Here's the drawing with two shaded views (mm, measured from the low corner). I have some questions. A direction names the side the tool comes from. Coordinates: 2 decimals unless noted, no trailing zeros. Order: outer loops, then holes, each group sorted by start corner. A loop starts at its lowest first (then second) coordinate and runs counter-clockwise, first axis right, second up. Notation, with made-up numbers: (-29.5, -35.75) -> (-23.5, -35.75) arc R31 cw to (-23.5, -4.75) -> close; hole circle Ø5 at (61.5, 20.25). An arc over 180 degrees is marked (long way). One line per item, written item: value. Start each with the question number.
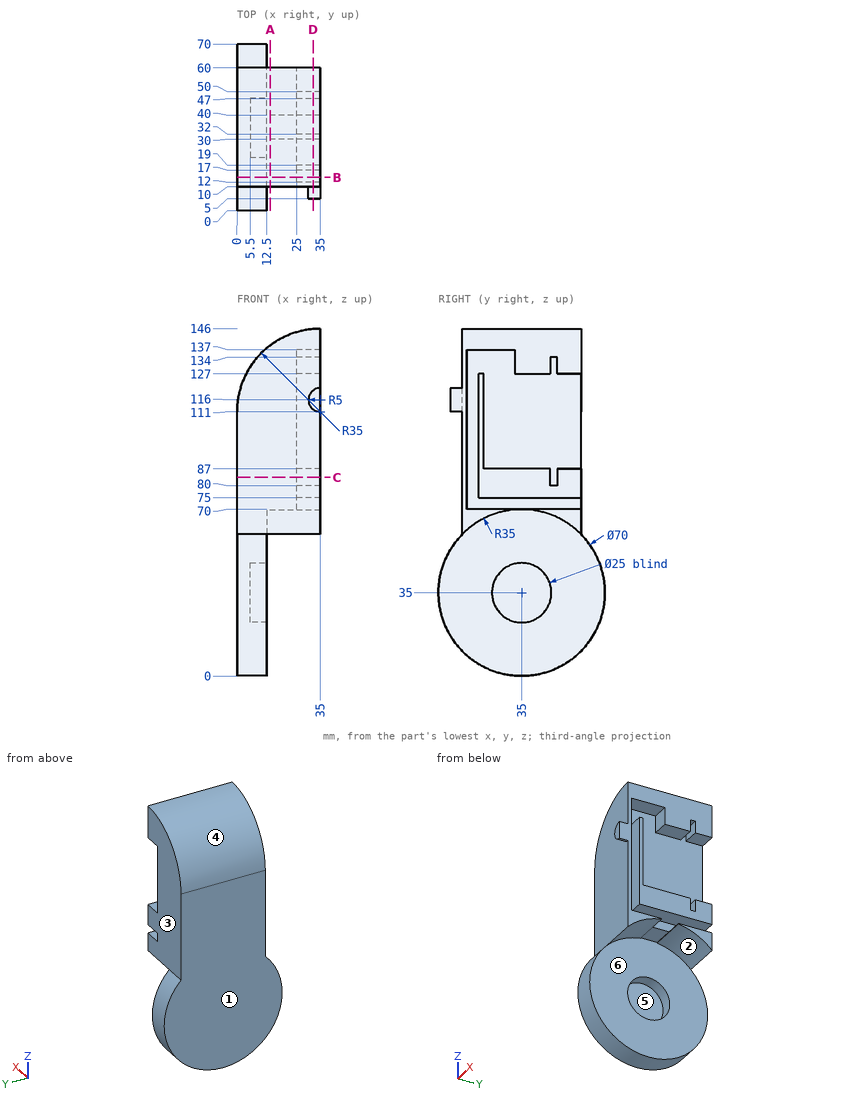
Q1. Imagine slicing it at C-C (z = 83.5). Write out the boundary of the cut face in (x, y), plus the area to 3 significant figures.
Q2. Imagine slicing it at A-A (x = 14). Write out the boundary of the cut face in (y, z), plus the area to 3 significant figures.
Q3. Imagine slicing it at B-B (y = 14). Write out the boundary of the cut face in (x, z), plus the area to 3 significant figures.
Q4. I need wall thicknesses on line 1 (Y direction, x = 33, z = 86.5); line 2 (Y direction, x = 31, z = 128); line 3 (Z direction, x = 33, y = 45). Which ranges of each line are inside material? Lowest first, please.
Q5. For P1, Ø3.5, axis at x = 29.5, z = 129, coming from the +Y side; P2, Ø5, axis at x = 28.5, z = 108, coming from the +Y side; P3, Ø1.5, axis at x = 31.5, z = 116, coming from the -Y side; P4, Ø12, axis at x = 20.5, z = 33.5, coming from the -Y side, each with a flat end and sliding along its axis, tell me the tip position at first contact or that it passes through.
Q6. For the marked faces 1, 2 and 3, which set-ups out of +Z, -Z, +X, -X, +Y, -Y let a thin tool reach every point of the face, with its end or its side?
Q7. If we mould it in two halves opening along Z, with no side actions, what happens to the marked faces 4, 5 and 6? For each: +Z half, -Z half, draft (parallel to the pull), parting line (faces both ways), or undercut.
Q8. Imagine slicing it at D-D (x = 32). Count the separate pieces of the cut face and the enclosed holes in it, plus the area to 3 significant figures.
Completed:
1. outline: (0, 10) -> (35, 10) -> (35, 12) -> (25, 12) -> (25, 17) -> (35, 17) -> (35, 47) -> (25, 47) -> (25, 50) -> (35, 50) -> (35, 60) -> (0, 60) -> close
1. area: 1,670 mm2
2. outline: (10, 59.49) arc R35 cw to (30, 69.64) -> (30, 70) -> (40, 70) -> (40, 69.64) arc R35 cw to (60, 59.49) -> (60, 139) -> (10, 139) -> close
2. area: 3,610 mm2
3. outline: (0, 7) -> (12.5, 7) -> (12.5, 63) -> (35, 63) -> (35, 70) -> (25, 70) -> (25, 137) -> (35, 137) -> (35, 146) arc R35 ccw to (0, 111) -> close
3. area: 2,670 mm2
4. line 1: y = 10 to 12, 17 to 47, 50 to 60
4. line 2: y = 10 to 12, 32 to 47, 50 to 60
4. line 3: z = 68.54 to 70, 75 to 87, 127 to 145.94
5. P1: stops at y = 60
5. P2: stops at y = 19
5. P3: stops at y = 5
5. P4: passes through
6. face 1: +Z, -Z, -X, +Y, -Y
6. face 2: -Z, +X
6. face 3: +Z, +X, -X, +Y
7. face 4: +Z half
7. face 5: undercut
7. face 6: draft
8. separate pieces: 3
8. enclosed holes: 0
8. area: 1,610 mm2
